Design review of the part built by this model. Coordinates are the model's own, in mm. A direction names the side the tool comes from. Coordinates: 2 decimals unless noted, no trailing zeros. Write each loop counter-clockwise with the first axis right and the second up, starting at its lowest first coordinate (ties: lowest second). Pieces come first, ordered by that corner, then holes. Notation, with made-up numbers: (8.5, 57.25) - (54.5, 57.25) arc R22 ccw to (54.5, 93.25) - close; hole circle Ø9 at (62, 4). An arc over 180 degrees is marked (long way). One line per item, written item: value.
from build123d import *

# Parameters (mm, degrees)
SKETCH_1_W      = 2
SKETCH_1_H      = 212
EXTRUDE_1_DEPTH = 1
FILLET_1_R      = 1
EXTRUDE_2_DEPTH = 1
FILLET_2_R      = 4


with BuildPart() as part:
    # Эскиз1 → Бобышка-Вытянуть1 (new body)
    with BuildSketch(Plane.XY):
        Polygon((3.5, 0), (16.5, 0), (16.5, 222), (3.5, 222), (3.5, 262), (0, 262), (0, 222), (0, 0), (0, -40), (3.5, -40), align=None)
        with Locations((9.5, 111)):
            Rectangle(SKETCH_1_W, SKETCH_1_H, mode=Mode.SUBTRACT)
    extrude(amount=EXTRUDE_1_DEPTH)

    # Скругление1
    fillet_1_edges = [part.edges().sort_by_distance(p)[0] for p in [
        (8.5, 5, 0.5),
        (10.5, 5, 0.5),
        (10.5, 217, 0.5),
        (8.5, 217, 0.5),
    ]]
    fillet(fillet_1_edges, radius=FILLET_1_R - 0.0001)  # a hair under: the kernel refuses the full size

    # Эскиз2 → Бобышка-Вытянуть2 (add)
    with BuildSketch(Plane.ZY):
        Polygon((0, -40), (28, -40), (28, -4), (15, -4), (15, 226), (28, 226), (28, 262), (0, 262), align=None)
    extrude(amount=-EXTRUDE_2_DEPTH)

    # Скругление2
    fillet_2_edges = [part.edges().sort_by_distance(p)[0] for p in [
        (0.5, 226, 15),
        (0.5, -4, 15),
    ]]
    fillet(fillet_2_edges, radius=FILLET_2_R)


solid = part.part
1. Consider section B-B, the plane z = 23. Write out the cut boundary in (x, y).
Answer block:
outline: (0, -40) - (1, -40) - (1, -4) - (0, -4) - close; (0, 226) - (1, 226) - (1, 262) - (0, 262) - close
2. Consider section D-D, the plane z = 7. Write out the cut boundary in (x, y).
Answer block:
outline: (0, -40) - (1, -40) - (1, 262) - (0, 262) - close
3. Consider section A-A, the plane y = 202. Write out the cut boundary in (x, z), then the cut area to 3 significant figures.
Answer block:
outline: (0, 0) - (8.5, 0) - (8.5, 1) - (1, 1) - (1, 15) - (0, 15) - close; (10.5, 0) - (16.5, 0) - (16.5, 1) - (10.5, 1) - close
area: 28.5 mm^2
4. Consider section C-C, the plane y = -14. Write out the cut boundary in (x, z).
Answer block:
outline: (0, 0) - (3.5, 0) - (3.5, 1) - (1, 1) - (1, 28) - (0, 28) - close
5. Wall thickness on line 1 along X through (y, z) = (131, 14): over which ranges is the line inside the solid? List them lowest first.
Answer block:
line 1: x = 0 to 1
6. For faces 1 (the face through (1, 113, 11)), 2 (the face through (0, 113, 11)), list the 3-axis set-ups (+Z, -Z, +X, -X, +Y, -Y) from which the entire face can be reached by the end or side of a thin tool; tool diameter is ignored.
Answer block:
face 1: +Z, +X, +Y, -Y
face 2: +Z, -Z, -X, +Y, -Y
7. Insertion check: pin 1 Ø8 at (y, z) = (88.5, 20.5) entering from +X; pin 2 Ø0.8 at (y, z) = (110, 0.5) entering from -X; pin 3 Ø0.5 at (x, z) = (13, 0.5) entering from -Y; pin 4 Ø1.5 at (x, y) = (14.5, 96) entering from +Z. Each pin has a flat end and moves straight along its axis. Give the tip position at first contact, or say it passes through.
Answer block:
pin 1: passes through
pin 2: stops at x = 0
pin 3: stops at y = 0
pin 4: stops at z = 1
